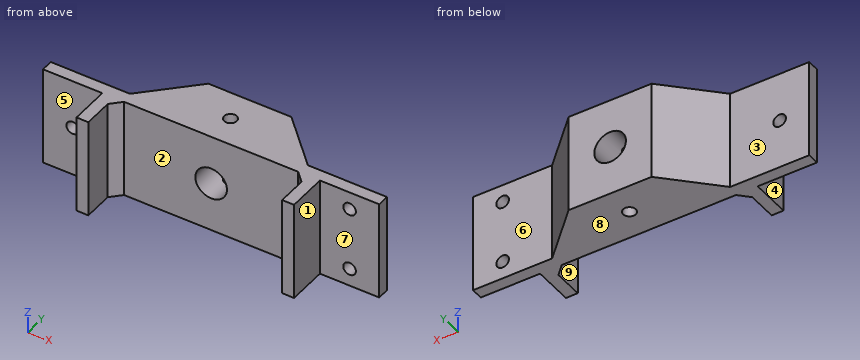
from build123d import *

# Parameters (mm, degrees)
SKETCH_1_W          = 85
SKETCH_1_H          = 3
EXTRUDE_1_DEPTH     = 25
SKETCH_2_W          = 3
SKETCH_2_H          = 25
EXTRUDE_2_DEPTH     = 10
SKETCH_3_W          = 3
SKETCH_3_H          = 25
EXTRUDE_3_DEPTH     = 10
SKETCH_4_W          = 25
SKETCH_4_H          = 25
EXTRUDE_1_2_DEPTH   = 12
CUT_EXTRUDE_1_REACH = 27
SKETCH_5_R          = 4
CHAMFER_1_SIZE      = 10
CHAMFER_2_SIZE      = 10
CUT_EXTRUDE_3_REACH = 27
CUT_EXTRUDE_4_REACH = 17
SKETCH_8_R          = 1.6
CHAMFER_4_SIZE      = 2.5
CHAMFER_5_SIZE      = 2.5
SKETCH_9_R          = 1.6
CUT_EXTRUDE_5_DEPTH = 25


with BuildPart() as part:
    # 草图1 → Extrude 1 (new body)
    with BuildSketch(Plane.XY):
        with Locations((0, -1.5)):
            Rectangle(SKETCH_1_W, SKETCH_1_H)
    extrude(amount=EXTRUDE_1_DEPTH)

    # 草图2 → 拉伸-薄壁2 (add)
    with BuildSketch(Plane.XZ.offset(3)):
        with Locations((-26, 12.5)):
            Rectangle(SKETCH_2_W, SKETCH_2_H)
    extrude(amount=EXTRUDE_2_DEPTH)

    # 草图3 → 拉伸-薄壁3 (add)
    with BuildSketch(Plane.XZ.offset(3)):
        with Locations((26, 12.5)):
            Rectangle(SKETCH_3_W, SKETCH_3_H)
    extrude(amount=EXTRUDE_3_DEPTH)

    # 草图4 → Extrude 1 2 (add)
    with BuildSketch(Plane(origin=(0, 0, 0), x_dir=(1, 0, 0), z_dir=(0, 1, 0))):
        with Locations((0, -12.5)):
            Rectangle(SKETCH_4_W, SKETCH_4_H)
    extrude(amount=EXTRUDE_1_2_DEPTH)

    # 草图5 → 切除-拉伸1 (cut, up to next)
    with BuildSketch(Plane(origin=(0, 12, 0), x_dir=(1, 0, 0), z_dir=(0, 1, 0)), mode=Mode.PRIVATE) as cut_extrude_1_sk1:
        with Locations((0, -12.5)):
            Circle(SKETCH_5_R)
    cut_extrude_1_tool1 = extrude(cut_extrude_1_sk1.sketch, amount=-CUT_EXTRUDE_1_REACH, mode=Mode.PRIVATE) & part.part
    add(cut_extrude_1_tool1.solids().sort_by_distance((0, 12, 12.5))[0], mode=Mode.SUBTRACT)

    # 倒角1
    chamfer_1_edges = [part.edges().sort_by_distance(p)[0] for p in [
        (12.5, 0, 12.5),
    ]]
    chamfer(chamfer_1_edges, length=CHAMFER_1_SIZE)

    # 倒角2
    chamfer_2_edges = [part.edges().sort_by_distance(p)[0] for p in [
        (-12.5, 0, 12.5),
    ]]
    chamfer(chamfer_2_edges, length=CHAMFER_2_SIZE)

    # 草图7 → 切除-拉伸3 (cut, up to next)
    with BuildSketch(Plane(origin=(0, 0, 0), x_dir=(-1, 0, 0), z_dir=(0, 0, -1)), mode=Mode.PRIVATE) as cut_extrude_3_sk1:
        Polygon((-12.5, 10), (-10.5, 12), (-12.5, 12), align=None)
    cut_extrude_3_tool1 = extrude(cut_extrude_3_sk1.sketch, amount=-CUT_EXTRUDE_3_REACH, mode=Mode.PRIVATE) & part.part
    add(cut_extrude_3_tool1.solids().sort_by_distance((11.833333, 11.333333, 0))[0], mode=Mode.SUBTRACT)
    # 草图7 → 切除-拉伸3 (cut, up to next)
    with BuildSketch(Plane(origin=(0, 0, 0), x_dir=(-1, 0, 0), z_dir=(0, 0, -1)), mode=Mode.PRIVATE) as cut_extrude_3_sk2:
        Polygon((12.5, 10), (10.5, 12), (12.5, 12), align=None)
    cut_extrude_3_tool2 = extrude(cut_extrude_3_sk2.sketch, amount=-CUT_EXTRUDE_3_REACH, mode=Mode.PRIVATE) & part.part
    add(cut_extrude_3_tool2.solids().sort_by_distance((-11.833333, 11.333333, 0))[0], mode=Mode.SUBTRACT)

    # 草图8 → 切除-拉伸4 (cut, up to next)
    with BuildSketch(Plane.XZ.offset(3), mode=Mode.PRIVATE) as cut_extrude_4_sk1:
        with Locations((35, 4.5)):
            Circle(SKETCH_8_R)
    cut_extrude_4_tool1 = extrude(cut_extrude_4_sk1.sketch, amount=-CUT_EXTRUDE_4_REACH, mode=Mode.PRIVATE) & part.part
    add(cut_extrude_4_tool1.solids().sort_by_distance((35, -3, 4.5))[0], mode=Mode.SUBTRACT)
    # 草图8 → 切除-拉伸4 (cut, up to next)
    with BuildSketch(Plane.XZ.offset(3), mode=Mode.PRIVATE) as cut_extrude_4_sk2:
        with Locations((35, 20.5)):
            Circle(SKETCH_8_R)
    cut_extrude_4_tool2 = extrude(cut_extrude_4_sk2.sketch, amount=-CUT_EXTRUDE_4_REACH, mode=Mode.PRIVATE) & part.part
    add(cut_extrude_4_tool2.solids().sort_by_distance((35, -3, 20.5))[0], mode=Mode.SUBTRACT)
    # 草图8 → 切除-拉伸4 (cut, up to next)
    with BuildSketch(Plane.XZ.offset(3), mode=Mode.PRIVATE) as cut_extrude_4_sk3:
        with Locations((-35, 12.5)):
            Circle(SKETCH_8_R)
    cut_extrude_4_tool3 = extrude(cut_extrude_4_sk3.sketch, amount=-CUT_EXTRUDE_4_REACH, mode=Mode.PRIVATE) & part.part
    add(cut_extrude_4_tool3.solids().sort_by_distance((-35, -3, 12.5))[0], mode=Mode.SUBTRACT)

    # 倒角4
    chamfer_4_edges = [part.edges().sort_by_distance(p)[0] for p in [
        (24.5, -3, 12.5),
    ]]
    chamfer(chamfer_4_edges, length=CHAMFER_4_SIZE)

    # 倒角5
    chamfer_5_edges = [part.edges().sort_by_distance(p)[0] for p in [
        (-24.5, -3, 12.5),
    ]]
    chamfer(chamfer_5_edges, length=CHAMFER_5_SIZE)

    # 草图9 → 切除-拉伸5 (cut)
    with BuildSketch(Plane.XY.offset(25)):
        with Locations((0, 4.5)):
            Circle(SKETCH_9_R)
    extrude(amount=-CUT_EXTRUDE_5_DEPTH, mode=Mode.SUBTRACT)


solid = part.part
Read the model definition and answer for the solid it produces. Units are mm, in the model's axes. Face numbers are marked on the shaded views. A direction names the side the tool comes from. Coordinates: 2 decimals unless noted, no trailing zeros. Order: outer loops, then holes, each group sorted by start corner. A loop starts at its lowest first (then second) coordinate and runs counter-clockwise, first axis right, second up. Notation, with made-up numbers: (-36, 42.5) - (7, 42.5) arc R6 ccw to (7, 48.5) - close; hole circle Ø1 at (36, 69). An arc over 180 degrees is marked (long way). Use one line per item in the form item = value.
(1) For a pull along X with two mould halves and no side action, classify the marked faces 1, 2, 3 and 4 as pulls with the +X half, pulls with the -X half, needs draft (parallel to the pull), parting line crosses it, or undercut.
Computed values:
face_1 = pulls with the +X half
face_2 = undercut
face_3 = needs draft
face_4 = pulls with the -X half
(2) Section A-A, the plane z = 20.5 is taken. Give the vertices of the cut face in (x, y).
Computed values:
outline = (-42.5, -3) - (-27.5, -3) - (-27.5, -13) - (-24.5, -13) - (-24.5, -5.5) - (-22, -3) - (22, -3) - (24.5, -5.5) - (24.5, -13) - (27.5, -13) - (27.5, -3) - (33.4, -3) - (33.4, 0) - (22.5, 0) - (10.5, 12) - (-10.5, 12) - (-22.5, 0) - (-42.5, 0) - close; (36.6, -3) - (42.5, -3) - (42.5, 0) - (36.6, 0) - close; hole circle Ø3.2 at (0, 4.5)
(3) Given pin 1 Ø3.5 at (x, z) = (35, 4.5) entering from -Y; pin 2 Ø2.5 at (x, y) = (0, 4.5) entering from +Z; pin 3 Ø8 at (y, z) = (-9, 13.5) entering from -X; pin 4 Ø5 at (x, z) = (-21.5, 22.5) entering from +Y, each flat-ended and moving along its own axis, determine where each tip first touches the part or whether it passes through.
Computed values:
pin_1 = -3
pin_2 = through
pin_3 = -27.5
pin_4 = 3.5
(4) Section C-C, the plane z = 12.5 is taken. Give the vertices of the cut face in (x, y).
Computed values:
outline = (-42.5, -3) - (-36.6, -3) - (-36.6, 0) - (-42.5, 0) - close; (-33.4, -3) - (-27.5, -3) - (-27.5, -13) - (-24.5, -13) - (-24.5, -5.5) - (-22, -3) - (-4, -3) - (-4, 12) - (-10.5, 12) - (-22.5, 0) - (-33.4, 0) - close; (4, -3) - (22, -3) - (24.5, -5.5) - (24.5, -13) - (27.5, -13) - (27.5, -3) - (42.5, -3) - (42.5, 0) - (22.5, 0) - (10.5, 12) - (4, 12) - close
(5) Section B-B, the plane y = 4.5 is taken. Give the vertices of the cut face in (x, z), then the cut area to 3 significant figures.
Computed values:
outline = (-18, 0) - (-1.6, 0) - (-1.6, 8.83) arc R4 cw to (-1.6, 16.17) - (-1.6, 25) - (-18, 25) - close; (1.6, 0) - (18, 0) - (18, 25) - (1.6, 25) - (1.6, 16.17) arc R4 cw to (1.6, 8.83) - close
area = 795 mm²
(6) Section D-D, the plane x = -35 is taken. Give the vertices of the cut face in (y, z), then the cut area to 3 significant figures.
Computed values:
outline = (-3, 0) - (0, 0) - (0, 10.9) - (-3, 10.9) - close; (-3, 14.1) - (0, 14.1) - (0, 25) - (-3, 25) - close
area = 65.4 mm²
(7) Straight lines are drawn through the part: L1, parallel to Y at x = 0, z = 19.75; L2, parallel to X at y = -6.75, z = 1; L3, parallel to Z at x = -35, y = -0.9. For each, find the intervals that lie inside material, in ascending order.
Computed values:
L1 = -3 to 2.9, 6.1 to 12
L2 = -27.5 to -24.5, 24.5 to 27.5
L3 = 0 to 10.9, 14.1 to 25
(8) Which of the six approach directions +Z, -Z, +X, -X, +Y, -Y give full straight-line access (tool end or side, diameter ignored) to the marked faces 5, 6, 7, 8 and 9?
Computed values:
face_5 = +Z, -Z, -X, -Y
face_6 = +Z, -Z, +X, +Y
face_7 = +Z, -Z, +X, -Y
face_8 = -Z, +X, -X, +Y, -Y
face_9 = +Z, -Z, -Y
